from build123d import *

# Parameters (mm, degrees)
F0_R     = 8.89
F1_DEPTH = 177.8
F2_W     = 50.8
F2_H     = 50.8
F3_DEPTH = 6.35
F5_DEPTH = 38.1


with BuildPart() as f1:
    # F0 (on Right) → F1 (new body)
    with BuildSketch(Plane.YZ):
        Circle(F0_R)
    extrude(amount=F1_DEPTH)

    # F2 (on Right) → F3 (join)
    with BuildSketch(Plane.YZ):
        Rectangle(F2_W, F2_H)
    extrude(amount=-F3_DEPTH)

    # F4 (on face) → F5 (join)
    with BuildSketch(Plane(origin=(-6.35, 0, 0), x_dir=(0, -1, 0), z_dir=(-1, 0, 0))):
        with BuildLine():
            ThreePointArc((6.286179, 6.286179), (11.822314, 5.184974), (14.958282, 9.878282))
            ThreePointArc((14.958282, 9.878282), (14.57159, 11.822314), (13.470384, 13.470384))
            Line((13.470384, 13.470384), (6.286179, 6.286179))
        make_face()
        with BuildLine():
            ThreePointArc((14.95827, -9.87827), (11.822302, -5.184962), (6.286168, -6.286168))
            Line((6.286168, -6.286168), (13.470373, -13.470373))
            ThreePointArc((13.470373, -13.470373), (14.571578, -11.822302), (14.95827, -9.87827))
        make_face()
        with BuildLine():
            Line((13.470373, -13.470373), (6.286168, -6.286168))
            ThreePointArc((6.286168, -6.286168), (6.286168, -13.470373), (13.470373, -13.470373))
        make_face()
        with BuildLine():
            ThreePointArc((-4.798282, -9.878282), (-5.184974, -7.93425), (-6.286179, -6.286179))
            Line((-6.286179, -6.286179), (-13.470384, -13.470384))
            ThreePointArc((-13.470384, -13.470384), (-7.93425, -14.57159), (-4.798282, -9.878282))
        make_face()
        with BuildLine():
            Line((-13.470384, -13.470384), (-6.286179, -6.286179))
            ThreePointArc((-6.286179, -6.286179), (-13.470384, -6.286179), (-13.470384, -13.470384))
        make_face()
        with BuildLine():
            ThreePointArc((-13.470396, 13.470396), (-13.470396, 6.286191), (-6.286191, 6.286191))
            Line((-6.286191, 6.286191), (-13.470396, 13.470396))
        make_face()
        with BuildLine():
            Line((-13.470396, 13.470396), (-6.286191, 6.286191))
            ThreePointArc((-6.286191, 6.286191), (-5.184985, 7.934262), (-4.798293, 9.878293))
            ThreePointArc((-4.798293, 9.878293), (-7.934262, 14.571601), (-13.470396, 13.470396))
        make_face()
        with BuildLine():
            Line((6.286179, 6.286179), (13.470384, 13.470384))
            ThreePointArc((13.470384, 13.470384), (6.286179, 13.470384), (6.286179, 6.286179))
        make_face()
    extrude(amount=F5_DEPTH)


solid = f1.part
Check sheet for the modelled part. Datum: model origin and axes. Units: mm. A direction names the side the tool comes from. Coordinates: 2 decimals unless noted, no trailing zeros. Loops run counter-clockwise (first coordinate to the right, second up) from the corner with the lowest first, then second, coordinate; pieces in that order, holes last. Notation, with made-up numbers: (-16.5, 43) -> (19.5, 43) arc R11 cw to (19.5, 63) -> close; hole circle Ø11 at (68, -12). An arc over 180 degrees is marked (long way). Write item = value, one per line. Start each with the question number.
1. Material ranges on line 1 (X direction, y = 6.5, z = -19.5); line 2 (X direction, y = -1.5, z = 3); line 3 (Z direction, x = 163, y = 0.5), recorded low to high.
2. Tool access check on faces 1 (the flat face through (0, 11, 0)), 2 (the flat face through (-3, 0, 25.4)), 3 (the flat face through (-6.35, 0, 0)). Record the directions out of +Z, -Z, +X, -X, +Y, -Y that give a thin tool (end or side, any length) a straight path to the whole face; none if there is none.
3. Section check A-A on y = 0. Record the cut outline in (x, z), then the cut area to 3 significant figures.
4. Section check D-D on z = -22. Record the cut outline in (x, y), then the cut area to 3 significant figures.
5. Section check C-C on x = 9.5. Record the cut outline in (y, z).
6. Depth check by flat-ended pin: P1, Ø4, axis at y = 0, z = 14.5, coming from the +X side; P2, Ø12, axis at x = 132, z = -11.5, coming from the -Y side; P3, Ø12, axis at x = 121, y = -7.5, coming from the -Z side. Enter the tip coordinate at first touch or a pass-through.
Responses:
q1.line_1 = -6.35 to 0
q1.line_2 = -6.35 to 177.8
q1.line_3 = -8.88 to 8.88
q2.face_1 = +X
q2.face_2 = +Z, +X, -X, +Y, -Y
q2.face_3 = -X
q3.outline = (-6.35, -25.4) -> (0, -25.4) -> (0, -8.89) -> (177.8, -8.89) -> (177.8, 8.89) -> (0, 8.89) -> (0, 25.4) -> (-6.35, 25.4) -> close
q3.area = 3,480 mm2
q4.outline = (-6.35, -25.4) -> (0, -25.4) -> (0, 25.4) -> (-6.35, 25.4) -> close
q4.area = 323 mm2
q5.outline = circle Ø17.78 at (0, 0)
q6.P1 = 0
q6.P2 = -6.98
q6.P3 = -8.76
